```python
from build123d import *

# Parameters (mm, degrees)
SKETCH1_R                = 40
BOSS_EXTRUDE1_DEPTH      = 6
SKETCH2_R                = 1.5
BOSS_EXTRUDE2_DEPTH      = 10
SKETCH16_R               = 1.5
CUT_EXTRUDE9_DEPTH       = 17
CIRPATTERN1_COUNT        = 3
SKETCH5_R                = 30.471270003
CUT_EXTRUDE3_DEPTH       = 7
CIRPATTERN2_COUNT        = 3
SKETCH17_W               = 12
SKETCH17_H               = 16
BOSS_EXTRUDE3_DEPTH      = 12
FILLET1_R                = 4
FILLET2_R                = 4
SKETCH18_R               = 4
CUT_EXTRUDE10_DEPTH      = 23.641777725
CUT_EXTRUDE10_DEPTH_BACK = 49


with BuildPart() as part:
    # Sketch1 → Boss-Extrude1 (new body)
    with BuildSketch(Plane(origin=(0, 0, 0), x_dir=(1, 0, 0), z_dir=(0, 1, 0))):
        Circle(SKETCH1_R)
    extrude(amount=BOSS_EXTRUDE1_DEPTH)

    # Sketch2 → Boss-Extrude2 (add)
    with BuildSketch(Plane(origin=(0, 6, 0), x_dir=(1, 0, 0), z_dir=(0, 1, 0))):
        with BuildLine():
            Line((-13.680805733, 37.587704831), (-10.944644586, 30.070163865))
            ThreePointArc((-10.944644586, 30.070163865), (0, 32), (10.944644586, 30.070163865))
            Line((10.944644586, 30.070163865), (13.680805733, 37.587704831))
            ThreePointArc((13.680805733, 37.587704831), (0, 40), (-13.680805733, 37.587704831))
        make_face()
        with Locations((0, 36)):
            Circle(SKETCH2_R, mode=Mode.SUBTRACT)
    boss_extrude2 = extrude(amount=BOSS_EXTRUDE2_DEPTH)

    # Sketch16 → Cut-Extrude9 (cut, through all)
    with BuildSketch(Plane(origin=(0, 16, 0), x_dir=(1, 0, 0), z_dir=(0, 1, 0))):
        with Locations((0, 36)):
            Circle(SKETCH16_R)
    cut_extrude9 = extrude(amount=-CUT_EXTRUDE9_DEPTH, mode=Mode.SUBTRACT)

    # CirPattern1: Boss-Extrude2, Cut-Extrude9 ×3 about axis
    cirpattern1_axis = Axis((0, 0, 0), (0, 1, 0))
    for i in range(1, CIRPATTERN1_COUNT):
        add(boss_extrude2.rotate(cirpattern1_axis, i * 360 / CIRPATTERN1_COUNT))
        add(cut_extrude9.rotate(cirpattern1_axis, i * 360 / CIRPATTERN1_COUNT), mode=Mode.SUBTRACT)

    # Sketch5 → Cut-Extrude3 (cut, through all)
    with BuildSketch(Plane(origin=(0, 6, 0), x_dir=(1, 0, 0), z_dir=(0, 1, 0))):
        with Locations((40.698571494, 23.497331208)):
            Circle(SKETCH5_R)
    cut_extrude3 = extrude(amount=-CUT_EXTRUDE3_DEPTH, mode=Mode.SUBTRACT)

    # CirPattern2: Cut-Extrude3 ×3 about axis
    cirpattern2_axis = Axis((0, 0, 0), (0, 1, 0))
    for i in range(1, CIRPATTERN2_COUNT):
        add(cut_extrude3.rotate(cirpattern2_axis, i * 360 / CIRPATTERN2_COUNT), mode=Mode.SUBTRACT)

    # Sketch17 → Boss-Extrude3 (add)
    with BuildSketch(Plane.XZ):
        Rectangle(SKETCH17_W, SKETCH17_H)
    extrude(amount=BOSS_EXTRUDE3_DEPTH)

    # Fillet1
    fillet1_edges = [part.edges().sort_by_distance(p)[0] for p in [
        (-6, 0, 0),
        (6, 0, 0),
        (-6, -12, 0),
        (6, -12, 0),
    ]]
    fillet(fillet1_edges, radius=FILLET1_R)

    # Fillet2
    fillet2_edges = [part.edges().sort_by_distance(p)[0] for p in [
        (0, 0, 8),
        (0, 0, -8),
    ]]
    fillet(fillet2_edges, radius=FILLET2_R)

    # Sketch18 → Cut-Extrude10 (cut, two sides)
    with BuildSketch(Plane.XY.offset(8)) as cut_extrude10_sk:
        with Locations((0, -6)):
            Circle(SKETCH18_R)
    extrude(amount=CUT_EXTRUDE10_DEPTH, mode=Mode.SUBTRACT)
    extrude(cut_extrude10_sk.sketch, amount=-CUT_EXTRUDE10_DEPTH_BACK, mode=Mode.SUBTRACT)


solid = part.part
```
For this review, take the finished solid that the model builds, in its own axes (mm). A direction names the side the tool comes from. Coordinates: 2 decimals unless noted, no trailing zeros. Write each loop counter-clockwise with the first axis right and the second up, starting at its lowest first coordinate (ties: lowest second). Pieces come first, ordered by that corner, then holes. Notation, with made-up numbers: (23.5, -2) - (79.5, -2) arc R34 cw to (79.5, 29) - close; hole circle Ø4 at (-19, 75.25). An arc over 180 degrees is marked (long way). Put each result on its own line as item: value.
1. Add section C-C, the plane z = 18. Give the boundary of the cut face in (x, y).
Values found:
outline: (-35.72, 0) - (-32.68, 0) - (-32.68, 16) - (-35.72, 16) - close; (-29.68, 0) - (-9.37, 0) - (-9.37, 6) - (-26.46, 6) - (-26.46, 16) - (-29.68, 16) - close; (9.37, 0) - (29.68, 0) - (29.68, 16) - (26.46, 16) - (26.46, 6) - (9.37, 6) - close; (32.68, 0) - (35.72, 0) - (35.72, 16) - (32.68, 16) - close
2. Add section A-A, the plane y = 7. Give the boundary of the cut face in (x, z), then the cut area to 3 significant figures.
Values found:
outline: (-39.39, 6.95) - (-31.51, 5.56) arc R32 cw to (-20.57, 24.51) - (-25.71, 30.64) arc R40 ccw to start; (-13.68, -37.59) arc R40 ccw to (13.68, -37.59) - (10.94, -30.07) arc R32 cw to (-10.94, -30.07) - close; (20.57, 24.51) arc R32 cw to (31.51, 5.56) - (39.39, 6.95) arc R40 ccw to (25.71, 30.64) - close; hole circle Ø3 at (-31.18, 18); hole circle Ø3 at (0, -36); hole circle Ø3 at (31.18, 18)
area: 582 mm²
3. Add section D-D, the plane z = -6. Give the boundary of the cut face in (x, y).
Values found:
outline: (-15.75, 0) - (-10, 0) arc R4 cw to (-6, -4) - (-6, -8) arc R4 ccw to (-2, -12) - (2, -12) arc R4 ccw to (6, -8) - (6, -4) arc R4 cw to (10, 0) - (15.75, 0) - (15.75, 6) - (-15.75, 6) - close; hole circle Ø8 at (0, -6)
4. Add section B-B, the plane x = 0. Give the boundary of the cut face in (y, z).
Values found:
outline: (-12, -8) - (-10, -8) - (-10, 8) - (-12, 8) - close; (-2, -8.54) arc R4 cw to (0, -12) - (0, -34.5) - (16, -34.5) - (16, -32) - (6, -32) - (6, 16.52) - (0, 16.52) - (0, 12) arc R4 cw to (-2, 8.54) - close; (0, -40) - (16, -40) - (16, -37.5) - (0, -37.5) - close
5. For pin 1 (3 mm diameter, centred on x = -3, y = 8.5, fed in from +Z); pin 2 (17 mm diameter, centred on x = 14, z = -0.5, fed in from +Y); pin 3 (4 mm diameter, centred on x = -31.18, z = 18, fed in from +Y); pin 4 (1.2 mm diameter, centred on y = -6.5, z = -2.5, fed in from -X), all flat-tipped, find the tip position at first contact; note any pin that passes through.
Values found:
pin 1: z = -31.68
pin 2: y = 6
pin 3: y = 16
pin 4: x = -6
6. Machinability: for faces 4 (the flat face through (0, -12, 0)), 5 (the flat face through (-6, -6, 0)), 6 (the flat face through (-23.176, 10.93, 27.62)), which of the approach directions +Z, -Z, +X, -X, +Y, -Y give a long, thin tool a straight path to every point of the face, cutting with its end or side? Answer none if there is none.
Values found:
face 4: +Z, -Z, +X, -X, -Y
face 5: +Z, -Z, -X, -Y
face 6: +Z, +Y, -Y
7. Wall thickness on probe 1 along X at (y, z) = (-6, -1.25); probe 2 along X at (y, z) = (12.5, 19); probe 3 along Y at (x, z) = (-6.5, -12.5): over which ranges is each line inside the solid? List them lowest first.
Values found:
probe 1: -6 to -4, 4 to 6
probe 2: -35.2 to -32.29, -30.06 to -25.75, 25.75 to 30.06, 32.29 to 35.2
probe 3: 0 to 6
8. Mouldability with a two-part tool opening along X and no side actions: class faces 1 (the cylindrical face through (14.1, 3.04, -8.63)), 2 (the flat face through (-29, 16, 17)), 3 (the flat face through (23.1, 10.93, 27.53)) as released by +X, released by -X, zero draft, split by the parting line, or undercut.
Values found:
face 1: released by +X
face 2: zero draft
face 3: undercut
